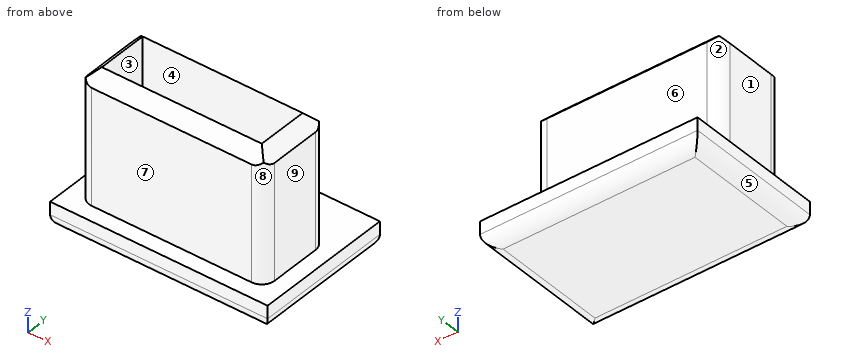
```python
from build123d import *

# Parameters (mm, degrees)
F0_W      = 34
F0_H      = 22
F1_DEPTH  = 4
F2_W      = 29
F2_H      = 12
F3_DEPTH  = 20
F4_SIZE   = 2
F3_FACE_W = 25
F3_FACE_H = 8
F5_DEPTH  = 20
F6_R      = 2
F7_R      = 2


with BuildPart() as f1:
    # F0 (on Top) → F1 (new body)
    with BuildSketch(Plane.XY):
        Rectangle(F0_W, F0_H)
    extrude(amount=F1_DEPTH)

    # F2 (on face) → F3 (join)
    with BuildSketch(Plane.XY.offset(4)):
        with Locations((0, -2.5)):
            Rectangle(F2_W, F2_H)
    extrude(amount=F3_DEPTH)

    # F4
    f4_edges = [f1.edges().sort_by_distance(p)[0] for p in [
        (0, 3.5, 24),
        (-14.5, -2.5, 24),
        (0, -8.5, 24),
        (14.5, -2.5, 24),
    ]]
    chamfer(f4_edges, length=F4_SIZE)

    # F3_face (on face) → F5 (cut)
    with BuildSketch(Plane(origin=(0, -2.5, 24), x_dir=(1, 0, 0), z_dir=(0, 0, 1))):
        Rectangle(F3_FACE_W, F3_FACE_H)
    extrude(amount=-F5_DEPTH, mode=Mode.SUBTRACT)

    # F6
    f6_edges = [f1.edges().sort_by_distance(p)[0] for p in [
        (0, -11, 0),
        (17, 0, 0),
        (-17, 0, 0),
        (0, 11, 0),
    ]]
    fillet(f6_edges, radius=F6_R)

    # F7
    f7_edges = [f1.edges().sort_by_distance(p)[0] for p in [
        (-14.5, -8.5, 13),
        (-14.5, 3.5, 13),
        (14.5, -8.5, 13),
        (14.5, 3.5, 13),
    ]]
    fillet(f7_edges, radius=F7_R)


solid = f1.part
```
Input: part model. Units: mm. Frame: model coordinates. Face numbers are marked on the shaded views. A direction names the side the tool comes from. Coordinates: 2 decimals unless noted, no trailing zeros. Loops run counter-clockwise (first coordinate to the right, second up) from the corner with the lowest first, then second, coordinate; pieces in that order, holes last. Notation, with made-up numbers: (69.5, 8.25) -> (116.5, 8.25) arc R24 ccw to (116.5, 21.25) -> close; hole circle Ø4 at (-12, 51). An arc over 180 degrees is marked (long way). Use a Markdown table: item, result.
1) Contact query for flat-ended pins moving along their axis: pin 1 (4 mm diameter, centred on y = -3, z = 16.5, fed in from +X); pin 2 (6 mm diameter, centred on x = 3, z = 15, fed in from -Y); pin 3 (6.5 mm diameter, centred on y = -1, z = 17, fed in from -X). Output: stop coordinate, or through.
Results found:
| item | result |
|---|---|
| pin 1 | stops at x = 14.5 |
| pin 2 | stops at y = -8.5 |
| pin 3 | stops at x = -14.5 |
2) Access query for the marked faces 5, 6, 7, 8 and 9. Directions: +Z, -Z, +X, -X, +Y, -Y. A direction counts if a zero-diameter tool reaches every point of the face in a straight line with its end or side. Return the directions, or none.
Results found:
| item | result |
|---|---|
| face 5 | -Z, -X, +Y, -Y |
| face 6 | +Z, +X, -X, +Y |
| face 7 | +Z, +X, -X, -Y |
| face 8 | +Z, +X, -Y |
| face 9 | +Z, +X, +Y, -Y |
3) Pull-direction query (Y, two-part tool) for the marked faces 1, 2, 3 and 4; classes: released by +Y, released by -Y, zero draft, split by the parting line, or undercut.
Results found:
| item | result |
|---|---|
| face 1 | zero draft |
| face 2 | released by +Y |
| face 3 | undercut |
| face 4 | undercut |
4) Material intervals for line 1 along X through (y, z) = (-5.5, 21.25); line 2 along Y through (x, z) = (-12, 11.5); line 3 along Z through (x, y) = (-9, 8.5), sorted ascending. Write a range as from..to.
Results found:
| item | result |
|---|---|
| line 1 | x = -14.5..-12.5, 12.5..14.5 |
| line 2 | y = -8.5..-6.5, 1.5..3.5 |
| line 3 | z = 0..4 |
5) Cut plane C-C (y = -1.75). Return the cut outline in (x, z), then the cut area to 3 significant figures.
Results found:
| item | result |
|---|---|
| outline | (-17, 2) arc R2 ccw to (-15, 0) -> (15, 0) arc R2 ccw to (17, 2) -> (17, 4) -> (14.5, 4) -> (14.5, 22) -> (12.5, 24) -> (12.5, 4) -> (-12.5, 4) -> (-12.5, 24) -> (-14.5, 22) -> (-14.5, 4) -> (-17, 4) -> close |
| area | 210 mm2 |
6) Cut plane B-B (x = 11). Return the cut outline in (y, z), then the cut area to 3 significant figures.
Results found:
| item | result |
|---|---|
| outline | (-11, 2) arc R2 ccw to (-9, 0) -> (9, 0) arc R2 ccw to (11, 2) -> (11, 4) -> (3.5, 4) -> (3.5, 22) -> (1.5, 24) -> (1.5, 4) -> (-6.5, 4) -> (-6.5, 24) -> (-8.5, 22) -> (-8.5, 4) -> (-11, 4) -> close |
| area | 162 mm2 |
7) Cut plane A-A (z = 20). Return the cut outline in (x, y), then the cut area to 3 significant figures.
Results found:
| item | result |
|---|---|
| outline | (-14.5, -6.5) arc R2 ccw to (-12.5, -8.5) -> (12.5, -8.5) arc R2 ccw to (14.5, -6.5) -> (14.5, 1.5) arc R2 ccw to (12.5, 3.5) -> (-12.5, 3.5) arc R2 ccw to (-14.5, 1.5) -> close; hole (-12.5, -6.5) -> (12.5, -6.5) -> (12.5, 1.5) -> (-12.5, 1.5) -> close |
| area | 145 mm2 |
8) Cut plane D-D (y = 2.5). Return the cut outline in (x, z), then the cut area to 3 significant figures.
Results found:
| item | result |
|---|---|
| outline | (-17, 2) arc R2 ccw to (-15, 0) -> (15, 0) arc R2 ccw to (17, 2) -> (17, 4) -> (14.23, 4) -> (14.23, 22.27) -> (13.5, 23) -> (-13.5, 23) -> (-14.23, 22.27) -> (-14.23, 4) -> (-17, 4) -> close |
| area | 675 mm2 |
